from build123d import *

# Parameters (mm, degrees)
FLEXURE_BOSS_DEPTH            = 5.18
SKETCH2_W                     = 10.5
SKETCH2_H                     = 18
SKETCH2_R                     = 1.575
MOUNTING_PLATE_BOSS_DEPTH     = 1.5
SKETCH7_W                     = 13
SKETCH7_H                     = 4.15
DOVETAIL_CONNECTION_CUT_DEPTH = 3.455
M3X0_5_TAPPED_HOLE1_D         = 2.5
FILLET1_R                     = 1


with BuildPart() as part:
    # Sketch1 → Flexure Boss (new body)
    with BuildSketch(Plane(origin=(0, 0, 0), x_dir=(0, 0, -1), z_dir=(1, 0, 0))):
        with BuildLine():
            ThreePointArc((2.743651747, -2.066915143), (3.036544966, -1.359808362), (3.743651747, -1.066915143))
            Line((3.743651747, -1.066915143), (8.368651984, -1.066915143))
            Line((8.368651984, -1.066915143), (8.368651984, 5.433084857))
            Line((8.368651984, 5.433084857), (-4.631348016, 5.433084857))
            Line((-4.631348016, 5.433084857), (-4.631348016, -1.066915143))
            Line((-4.631348016, -1.066915143), (-2.201142923, -1.066915143))
            ThreePointArc((-2.201142923, -1.066915143), (-1.494036142, -1.359808362), (-1.201142923, -2.066915143))
            Line((-1.201142923, -2.066915143), (-1.201142923, -10.691915143))
            Line((-1.201142923, -10.691915143), (2.673857314, -10.691915143))
            Line((2.673857314, -10.691915143), (2.673857314, -11.441915143))
            Line((2.673857314, -11.441915143), (-0.951142686, -11.441915143))
            ThreePointArc((-0.951142686, -11.441915143), (-1.658249467, -11.149021924), (-1.951142686, -10.441915143))
            Line((-1.951142686, -10.441915143), (-1.951142686, -1.566915143))
            Line((-1.951142686, -1.566915143), (-4.701142686, -1.566915143))
            Line((-4.701142686, -1.566915143), (-4.701142686, -12.316915143))
            ThreePointArc((-4.701142686, -12.316915143), (-4.994035905, -13.024021924), (-5.701142686, -13.316915143))
            Line((-5.701142686, -13.316915143), (-6.391348016, -13.316915143))
            Line((-6.391348016, -13.316915143), (-6.391348016, -19.646915143))
            Line((-6.391348016, -19.646915143), (-1.391348016, -19.646915143))
            Line((-1.391348016, -19.646915143), (-1.391348016, -18.146915143))
            Line((-1.391348016, -18.146915143), (-4.891348016, -18.146915143))
            Line((-4.891348016, -18.146915143), (-4.891348016, -14.816915143))
            Line((-4.891348016, -14.816915143), (-4.631348016, -14.816915143))
            Line((-4.631348016, -14.816915143), (15.425469929, -14.816915143))
            Line((15.425469929, -14.816915143), (15.425469929, -13.316915143))
            Line((15.425469929, -13.316915143), (14.743651747, -1.316915143))
            Line((14.743651747, -1.316915143), (11.993651747, -1.316915143))
            Line((11.993651747, -1.316915143), (11.993651747, -11.816915143))
            Line((11.993651747, -11.816915143), (11.743651747, -11.816915143))
            ThreePointArc((11.743651747, -11.816915143), (11.390098357, -11.670468534), (11.243651747, -11.316915143))
            Line((11.243651747, -11.316915143), (11.243651747, -1.816915143))
            Line((11.243651747, -1.816915143), (8.743651747, -1.816915143))
            Line((8.743651747, -1.816915143), (8.743651747, -2.316915143))
            Line((8.743651747, -2.316915143), (3.243651747, -2.316915143))
            Line((3.243651747, -2.316915143), (3.243651747, -4.816915143))
            Line((3.243651747, -4.816915143), (8.743651747, -4.816915143))
            Line((8.743651747, -4.816915143), (8.743651747, -5.316915143))
            ThreePointArc((8.743651747, -5.316915143), (8.670428443, -5.493691838), (8.493651747, -5.566915143))
            Line((8.493651747, -5.566915143), (2.743651747, -5.566915143))
            Line((2.743651747, -5.566915143), (2.743651747, -2.066915143))
        make_face()
        with BuildLine():
            ThreePointArc((-0.326142923, -9.316915143), (-0.252919618, -9.140138448), (-0.076142923, -9.066915143))
            Line((-0.076142923, -9.066915143), (9.548857077, -9.066915143))
            Line((9.548857077, -9.066915143), (9.548857077, -3.941915143))
            Line((9.548857077, -3.941915143), (4.243651747, -3.941915143))
            Line((4.243651747, -3.941915143), (4.243651747, -3.191915143))
            Line((4.243651747, -3.191915143), (9.298857077, -3.191915143))
            ThreePointArc((9.298857077, -3.191915143), (10.005963858, -3.484808362), (10.298857077, -4.191915143))
            Line((10.298857077, -4.191915143), (10.298857077, -12.816915143))
            Line((10.298857077, -12.816915143), (13.048857077, -12.816915143))
            Line((13.048857077, -12.816915143), (13.048857077, -2.316915143))
            Line((13.048857077, -2.316915143), (13.798857077, -2.316915143))
            Line((13.798857077, -2.316915143), (14.37882611, -12.524370125))
            ThreePointArc((14.37882611, -12.524370125), (14.175198347, -13.0819837), (13.630033801, -13.316915143))
            Line((13.630033801, -13.316915143), (-2.701142686, -13.316915143))
            ThreePointArc((-2.701142686, -13.316915143), (-3.408249467, -13.024021924), (-3.701142686, -12.316915143))
            Line((-3.701142686, -12.316915143), (-3.701142686, -2.566915143))
            Line((-3.701142686, -2.566915143), (-2.951142686, -2.566915143))
            Line((-2.951142686, -2.566915143), (-2.951142686, -12.816915143))
            Line((-2.951142686, -12.816915143), (-0.451142686, -12.816915143))
            Line((-0.451142686, -12.816915143), (-0.451142686, -12.316915143))
            Line((-0.451142686, -12.316915143), (3.673857314, -12.316915143))
            Line((3.673857314, -12.316915143), (3.673857314, -9.816915143))
            Line((3.673857314, -9.816915143), (-0.326142923, -9.816915143))
            Line((-0.326142923, -9.816915143), (-0.326142923, -9.316915143))
        make_face(mode=Mode.SUBTRACT)
    extrude(amount=FLEXURE_BOSS_DEPTH)

    # Sketch2 → Mounting Plate Boss (add)
    with BuildSketch(Plane.XZ.offset(14.816915143)):
        with Locations((-0.07, -16.309568548)):
            Rectangle(SKETCH2_W, SKETCH2_H)
        with Locations(Location((-2.435, -10.088651984, 0), (0, 0, 270))):
            Circle(SKETCH2_R, mode=Mode.SUBTRACT)
        with Locations(Location((-2.435, -22.088651984, 0), (0, 0, 270))):
            Circle(SKETCH2_R, mode=Mode.SUBTRACT)
    extrude(amount=-MOUNTING_PLATE_BOSS_DEPTH)

    # Sketch7 → Dovetail Connection Cut (cut)
    with BuildSketch(Plane.ZY):
        with Locations((-1.868651984, 2.508084857)):
            Rectangle(SKETCH7_W, SKETCH7_H)
    extrude(amount=-DOVETAIL_CONNECTION_CUT_DEPTH, mode=Mode.SUBTRACT)

    # M3x0.5 Tapped Hole1 (through all)
    with Locations(Plane(origin=(5.18, 0, 0), x_dir=(0, 0, -1), z_dir=(1, 0, 0))):
        with Locations((-1.381348016, 2.433084857), (5.118651984, 2.433084857)):
            Hole(M3X0_5_TAPPED_HOLE1_D / 2)


with BuildPart() as body_2:
    # Mirror2: mirrored copy
    add(part.part.mirror(Plane(origin=(5.18, 0, 0), x_dir=(0, 0, 1), z_dir=(1, 0, 0))))

    # Fillet1
    fillet1_edges = [body_2.edges().sort_by_distance(p)[0] for p in [
        (7.77, -13.316915143, -15.425469929),
    ]]
    fillet(fillet1_edges, radius=FILLET1_R)


solid = body_2.part
Verification items for the finished model (mm, model axes). A direction names the side the tool comes from. Coordinates: 2 decimals unless noted, no trailing zeros. Write each loop counter-clockwise with the first axis right and the second up, starting at its lowest first coordinate (ties: lowest second). Pieces come first, ordered by that corner, then holes. Notation, with made-up numbers: M 0,7.25 L 29,7.25 A24 ccw 29,29.25 Z; hole C 77,-37 d4. An arc over 180 degrees is marked long. Use a Markdown table: item, result.
Q1. Go/stop test with flat-tipped pins: P1, Ø1.6, axis at x = 7, z = -3, coming from the -Y side; P2, Ø4, axis at x = 14, y = 0, coming from the -Z side; P3, Ø4, axis at x = 7.5, y = -4, coming from the -Z side; P4, Ø1.2, axis at x = 8.5, y = -18.5, coming from the -Z side. Record where each tip stops, or that it passes through.
Reply:
| item | result |
|---|---|
| P1 | stops at y = -14.82 |
| P2 | passes through |
| P3 | stops at z = -15.01 |
| P4 | stops at z = 1.39 |
Q2. Set-up check for faces 4 (the face through (8, -1.817, -10)), 5 (the face through (9, 4.583, -2)), 6 (the face through (7.73, -13.05, -15.69)), 7 (the face through (8, -1.567, 3)), 8 (the face through (8, -8, 2.951)): record each of +Z, -Z, +X, -X, +Y, -Y from which the full face is reachable in a straight line by a thin tool's end or side.
Reply:
| item | result |
|---|---|
| face 4 | +X, -X, +Y |
| face 5 | +Z, -Z, +X |
| face 6 | -Z, +X, -X, +Y |
| face 7 | +Z, +X, -X |
| face 8 | +X, -X |
Q3. Sectioned sample at D-D, the plane y = 1.75. Record the boundary of the cut face in (x, z) (1 decimal).
Reply:
| item | result |
|---|---|
| outline | M 5.2,-8.4 L 6.9,-8.4 L 6.9,-6.2 L 5.2,-6.2 Z; M 5.2,-4.1 L 6.9,-4.1 L 6.9,0.3 L 5.2,0.3 Z; M 5.2,2.4 L 6.9,2.4 L 6.9,4.6 L 5.2,4.6 Z |
Q4. Sectioned sample at B-B, the plane x = 9. Count the separate pieces of the cut face and the enclosed holes in it, plus the area to 3 significant figures.
Reply:
| item | result |
|---|---|
| separate pieces | 2 |
| enclosed holes | 1 |
| area | 233 mm² |
Q5. Thickness scan on line 1 (Y direction, x = 7, z = -6); line 2 (Y direction, x = 7.5, z = -0.5); line 3 (Y direction, x = 6.5, z = -0.5). Record the ranges inside material, lowest first.
Reply:
| item | result |
|---|---|
| line 1 | y = -14.82 to -13.32, -9.07 to -5.57, -4.82 to -3.94, -3.19 to -2.32, -1.07 to 0.43, 4.58 to 5.43 |
| line 2 | y = -14.82 to -13.32, -12.32 to -11.44, -10.69 to -9.82, -9.07 to 0.43, 4.58 to 5.43 |
| line 3 | y = -14.82 to -13.32, -12.32 to -11.44, -10.69 to -9.82, -9.07 to 5.43 |
Q6. Sectioned sample at C-C, the plane z = -5. Record the boundary of the cut face in (x, y) (3 decimals), plus the area to 3 significant figures.
Reply:
| item | result |
|---|---|
| outline | M 5.18,-14.817 L 10.36,-14.817 L 10.36,-13.317 L 5.18,-13.317 Z; M 5.18,-9.067 L 10.36,-9.067 L 10.36,-5.567 L 5.18,-5.567 Z; M 5.18,-4.817 L 10.36,-4.817 L 10.36,-3.942 L 5.18,-3.942 Z; M 5.18,-3.192 L 10.36,-3.192 L 10.36,-2.317 L 5.18,-2.317 Z; M 5.18,-1.067 L 10.36,-1.067 L 10.36,0.433 L 6.905,0.433 L 6.905,1.189 L 5.18,1.189 Z; M 5.18,3.677 L 6.905,3.677 L 6.905,4.583 L 10.36,4.583 L 10.36,5.433 L 5.18,5.433 Z |
| area | 50.0 mm² |
Q7. Draft check along Y on faces 1 (the face through (7.806, -6.923, -15.062)), 2 (the face through (8, -7, 4.701)), 3 (the face through (8, -4, -2.744)). Enter one of: +Y half, -Y half, draft (parallel to the pull), parting line (faces both ways), or undercut.
Reply:
| item | result |
|---|---|
| face 1 | +Y half |
| face 2 | draft |
| face 3 | undercut |
Q8. Sectioned sample at A-A, the plane y = -7.75. Record the boundary of the cut face in (x, z), plus the area to 3 significant figures.
Reply:
| item | result |
|---|---|
| outline | M 5.18,-15.11 L 10.36,-15.11 L 10.36,-14.11 L 5.18,-14.11 Z; M 5.18,-13.05 L 10.36,-13.05 L 10.36,-11.99 L 5.18,-11.99 Z; M 5.18,-11.24 L 10.36,-11.24 L 10.36,-10.3 L 5.18,-10.3 Z; M 5.18,-9.55 L 10.36,-9.55 L 10.36,1.2 L 5.18,1.2 Z; M 5.18,1.95 L 10.36,1.95 L 10.36,2.95 L 5.18,2.95 Z; M 5.18,3.7 L 10.36,3.7 L 10.36,4.7 L 5.18,4.7 Z |
| area | 81.6 mm² |
